Can you work these out from the model? Positions are in its coordinate system, mm. Coordinates: 2 decimals unless noted, no trailing zeros. Order: outer loops, then holes, each group sorted by start corner. A loop starts at its lowest first (then second) coordinate and runs counter-clockwise, first axis right, second up. Notation, with made-up numbers: (35, 44.5) - (63, 44.5) arc R24 cw to (63, 72.5) - close; hole circle Ø11 at (32.25, 8.25). An arc over 180 degrees is marked (long way). Return JSON: item names as keys, results as strings. Group by question number.
1) Imagine slicing it at A-A (x = -48.5). Write out the boundary of the cut face in (y, z).
2) Imagine slicing it at B-B (y = 2.7). Write out the boundary of the cut face in (x, z), and give its area (3 significant figures).
3) If I drill on line 1 along Z through (x, y) = (27, 4.75); line 2 along X through (y, z) = (3.95, -4); line 3 along X through (y, z) = (3.2, -8), over which ranges is the centre line in solid material (lowest first)?
4) Imagine slicing it at C-C (z = -24). Write out the boundary of the cut face in (x, y).
5) Imagine slicing it at D-D (x = 15.5). Write out the boundary of the cut face in (y, z), and give its area (3 significant figures).
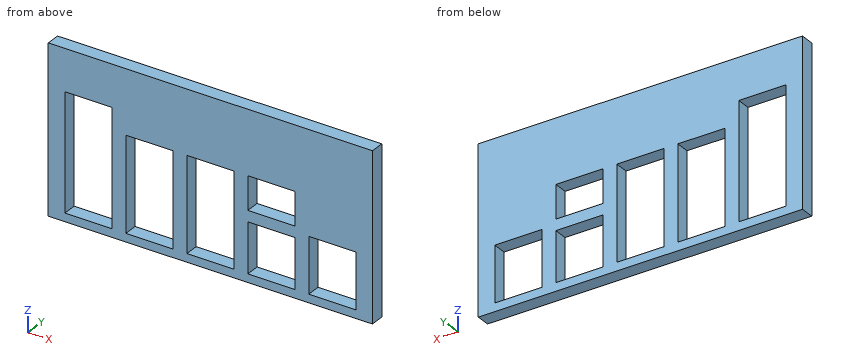
```python
from build123d import *

# Parameters (mm, degrees)
SKETCH1_W           = 117
SKETCH1_H           = 60
SKETCH1_W_2         = 17
SKETCH1_H_2         = 18
SKETCH1_H_3         = 42
SKETCH1_H_4         = 34
SKETCH1_H_5         = 20
SKETCH1_H_6         = 12
BOSS_EXTRUDE1_DEPTH = 5


with BuildPart() as part:
    # Sketch1 → Boss-Extrude1 (new body)
    with BuildSketch(Plane(origin=(0, 0, 0), x_dir=(1, 0, 0), z_dir=(0, 1, 0))):
        Rectangle(SKETCH1_W, SKETCH1_H)
        with Locations((22, 18)):
            Rectangle(SKETCH1_W_2, SKETCH1_H_2, mode=Mode.SUBTRACT)
        with Locations((-44, 6)):
            Rectangle(SKETCH1_W_2, SKETCH1_H_3, mode=Mode.SUBTRACT)
        with Locations((-22, 10)):
            Rectangle(SKETCH1_W_2, SKETCH1_H_4, mode=Mode.SUBTRACT)
        with Locations((0, 10)):
            Rectangle(SKETCH1_W_2, SKETCH1_H_4, mode=Mode.SUBTRACT)
        with Locations((44, 17)):
            Rectangle(SKETCH1_W_2, SKETCH1_H_5, mode=Mode.SUBTRACT)
        with Locations((22, -1)):
            Rectangle(SKETCH1_W_2, SKETCH1_H_6, mode=Mode.SUBTRACT)
    extrude(amount=BOSS_EXTRUDE1_DEPTH)


solid = part.part
```
Calculated:
{
 "1": {"outline": "(0, -30) - (5, -30) - (5, -27) - (0, -27) - close; (0, 15) - (5, 15) - (5, 30) - (0, 30) - close"},
 "2": {"outline": "(-58.5, -30) - (58.5, -30) - (58.5, 30) - (-58.5, 30) - close; hole (-52.5, -27) - (-35.5, -27) - (-35.5, 15) - (-52.5, 15) - close; hole (-30.5, -27) - (-13.5, -27) - (-13.5, 7) - (-30.5, 7) - close; hole (-8.5, -27) - (8.5, -27) - (8.5, 7) - (-8.5, 7) - close; hole (13.5, -27) - (30.5, -27) - (30.5, -9) - (13.5, -9) - close; hole (13.5, -5) - (30.5, -5) - (30.5, 7) - (13.5, 7) - close; hole (35.5, -27) - (52.5, -27) - (52.5, -7) - (35.5, -7) - close", "area": "4,300 mm2"},
 "3": {"line 1": "-30 to -27, -9 to -5, 7 to 30", "line 2": "-58.5 to -52.5, -35.5 to -30.5, -13.5 to -8.5, 8.5 to 13.5, 30.5 to 58.5", "line 3": "-58.5 to -52.5, -35.5 to -30.5, -13.5 to -8.5, 8.5 to 35.5, 52.5 to 58.5"},
 "4": {"outline": "(-58.5, 0) - (-52.5, 0) - (-52.5, 5) - (-58.5, 5) - close; (-35.5, 0) - (-30.5, 0) - (-30.5, 5) - (-35.5, 5) - close; (-13.5, 0) - (-8.5, 0) - (-8.5, 5) - (-13.5, 5) - close; (8.5, 0) - (13.5, 0) - (13.5, 5) - (8.5, 5) - close; (30.5, 0) - (35.5, 0) - (35.5, 5) - (30.5, 5) - close; (52.5, 0) - (58.5, 0) - (58.5, 5) - (52.5, 5) - close"},
 "5": {"outline": "(0, -30) - (5, -30) - (5, -27) - (0, -27) - close; (0, -9) - (5, -9) - (5, -5) - (0, -5) - close; (0, 7) - (5, 7) - (5, 30) - (0, 30) - close", "area": "150 mm2"}
}
